Could you check a few things on this model? Use its own coordinates, in mm. Face numbers are marked on the shaded views. A direction names the side the tool comes from. Coordinates: 2 decimals unless noted, no trailing zeros. Order: outer loops, then holes, each group sorted by start corner. A loop starts at its lowest first (then second) coordinate and runs counter-clockwise, first axis right, second up. Notation, with made-up numbers: (65, 82) - (109, 82) arc R30 ccw to (109, 105) - close; hole circle Ø3 at (7.5, 75.5). An arc over 180 degrees is marked (long way). One line per item, written item: value. Start each with the question number.
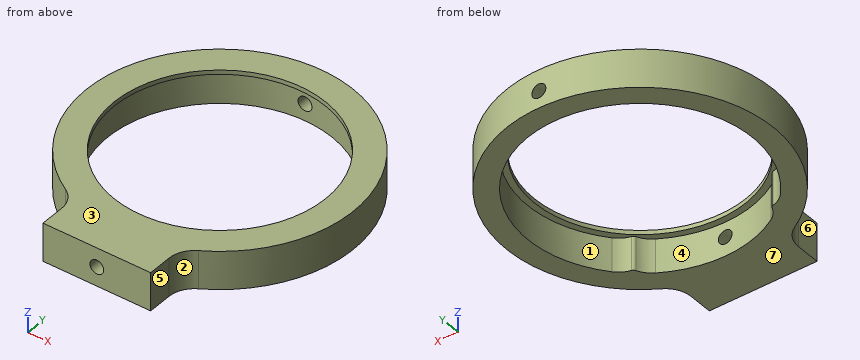
Autodesk Inventor part; units mm, degrees
ref_plane "Work Plane1" through (0, 31.4, 0) normal (0, 1, 0) x (-1, 0, 0)
ref_plane "YZ Plane" through (0, 0, 0) normal (1, 0, 0) x (0, 1, 0)
ref_plane "XY Plane" through (0, 0, 0) normal (0, 0, 1) x (1, 0, 0)
sketch "Sketch1" plane through (0, 0, 0) normal (0, 0, 1) x (1, 0, 0)
  circle A0 centre (0, 0) radius 25.4 construction
  circle A1 centre (0, 0) radius 26.4
  circle A2 centre (0, 0) radius 31.4
  line L0 (0, 0) -> (37.8275, -45.0811) construction
  line L1 (0, 0) -> (58.8492, 0) construction
  circle A3 centre (16.9696, -20.2236) radius 1
  line L2 (0, 0) -> (0, -31.4) construction
  circle A4 centre (-16.9696, -20.2236) radius 1
  dimension "d1" = 52.8
  dimension "d2" = 62.8
  dimension "d0" = 50.8
  dimension "d4" = 50
extrude "Extrusion1" add sketch "Sketch1" along normal blind 8 contours A4 A1 | A1 A4 | A3 A1 | A1 A3 | A2
fillet "Fillet1" radius 6 2 edges at (17.7233, -19.5664, 4) (16.1915, -20.8517, 4)
fillet_without_effect "Fillet2"
fillet "Fillet3" radius 6 2 edges at (-17.7233, -19.5664, 4) (-16.1915, -20.8517, 4)
fillet_without_effect "Fillet4"
sketch "Sketch2" plane through (0, 0, 8) normal (0, 0, 1) x (1, 0, 0)
  circle A0 centre (0, 0) radius 31.4
  arc A1 (19.8973, -17.351) -> (-19.8973, -17.351) centre (0, 0) ccw
  circle A2 centre (0, 0) radius 24.9
  circle A3 centre (0, 0) radius 31.4
  dimension "d11" = 49.8
extrude "Extrusion2" add sketch "Sketch2" along normal blind 1
ref_plane "Work Plane1" through (0, 31.4, 0) normal (0, 1, 0) x (-1, 0, 0)
sketch "Sketch3" plane through (0, 31.4, 0) normal (0, 1, 0) x (-1, 0, 0)
  line L0 (-31.4, 0) -> (31.4, 0)
  point P0 (0, 0)
  point P1 (0, 4)
  dimension "d14" = 4
hole "Hole1" at (0, 31.4, 4) direction (0, -1, 0) diameter 3.302 depth 12.3 tip angle 118
sketch "Sketch4" plane through (0, 0, 0) normal (0, 0, -1) x (-1, 0, 0)
  circle A0 centre (0, 0) radius 31.4
  arc A1 (-13.6322, -22.608) -> (13.6322, -22.608) centre (0, 0) ccw
  line L0 (-44.084, -38.1) -> (62.353, -38.1) construction
  line L1 (-12.7, -28.7171) -> (12.7, -28.7171)
  line L2 (12.7, -28.7171) -> (12.7, -38.1)
  line L3 (12.7, -38.1) -> (-12.7, -38.1)
  line L4 (-12.7, -38.1) -> (-12.7, -28.7171)
  line L5 (-12.7, -28.7171) -> (12.7, -38.1) construction
  line L6 (12.7, -28.7171) -> (-12.7, -38.1) construction
  line L7 (0, 0) -> (0, -74.2634) construction
  point P0 (0, -33.4085)
  point P1 (0, -33.4085)
  dimension "d22" = 38.1
  dimension "d23" = 25.4
extrude "Extrusion3" add sketch "Sketch4" against normal blind 9 contours L1 A0 | A0 L2 L3 L4 picked at (-2.1634, -29.3854)
fillet "Fillet5" radius 6 1 edges at (12.7, -28.7171, 4.5)
fillet "Fillet6" radius 6 1 edges at (-12.7, -28.7171, 4.5)
sketch "Sketch5" plane through (-12.7, -38.1, 0) normal (0, -1, 0) x (1, 0, 0)
  line L0 (0, 9) -> (25.4, 9)
  line L1 (0, 0) -> (0, 9)
  line L2 (12.7, 0) -> (12.7, 9) construction
  line L3 (25.4, 9) -> (25.4, 0) construction
  line L4 (25.4, 4.5) -> (0, 4.5) construction
  point P0 (12.7, 4.5)
hole "Hole2" at (0, -38.1, 4.5) direction (0, 1, 0) diameter 3.242 depth 13 tip angle 118
properties part number "BSholder"
Q1. I want a section at B-B on y = -7. Please give me the cut outline in (x, z).
Q2. I'm going to push flat-ended pins straight in: pin 1 (3 mm diameter, centred on x = -19.5, z = 8, fed in from -Y); pin 2 (2 mm diameter, centred on x = 10.5, y = -22.5, fed in from -Z); pin 3 (4.5 mm diameter, centred on y = -36.5, z = 4.5, fed in from +X). Where does each tip first touch, or does it pass through?
Q3. We'd pull the mould along Y, two halves only. Please class the marked faces 1, 2 and 3: +Y half, -Y half, draft (parallel to the pull), parting line (faces both ways), or undercut.
Q4. I want a section at A-A on y = 0. Please give me the cut outline in (x, z).
Q5. If I drill on L1, parallel to Z at x = 0, y = 29.5; L2, parallel to X at y = 0, z = 4.25; L3, parallel to X at y = 18.5, z = 2.75, over which ranges is the centre line in solid material (lowest first)?
Q6. Which directions (+Z, -Z, +X, -X, +Y, -Y) give clear straight access to the entire face, cutting with the end or side of a thin tool? Please do the marked faces 4, 5, 6 and 7.
Values follow:
1. outline: (-30.61, 0) - (-25.46, 0) - (-25.46, 8) - (-23.9, 8) - (-23.9, 9) - (-30.61, 9) - close; (23.9, 8) - (25.46, 8) - (25.46, 0) - (30.61, 0) - (30.61, 9) - (23.9, 9) - close
2. pin 1: stops at y = -25.73
2. pin 2: stops at z = 8
2. pin 3: stops at x = 12.7
3. face 1: undercut
3. face 2: -Y half
3. face 3: draft
4. outline: (-31.4, 0) - (-26.4, 0) - (-26.4, 8) - (-24.9, 8) - (-24.9, 9) - (-31.4, 9) - close; (24.9, 8) - (26.4, 8) - (26.4, 0) - (31.4, 0) - (31.4, 9) - (24.9, 9) - close
5. L1: z = 0 to 2.35, 5.65 to 9
5. L2: x = -31.4 to -26.4, 26.4 to 31.4
5. L3: x = -25.37 to -18.83, 18.83 to 25.37
6. face 4: -Z
6. face 5: +Z, -Z, +X, -Y
6. face 6: +Z, -Z, -X, -Y
6. face 7: -Z, +X, -X, +Y, -Y
